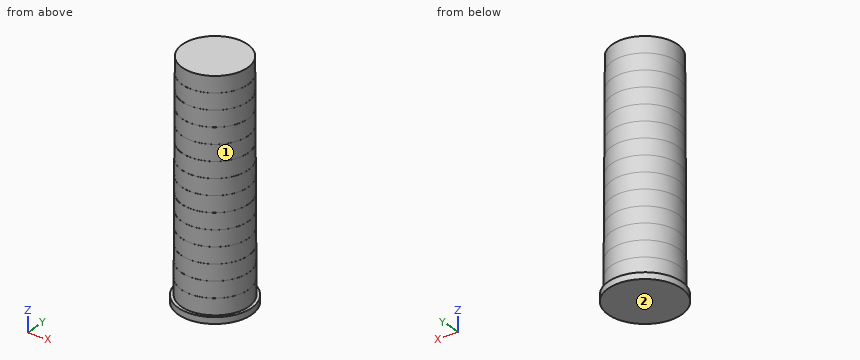
from build123d import *

# Parameters (mm, degrees)
F0_R      = 21.1
F1_DEPTH  = 10
F2_R      = 21.05
F3_DEPTH  = 10
F4_R      = 21
F5_DEPTH  = 10
F6_R      = 20.95
F7_DEPTH  = 10
F8_R      = 23
F8_R_2    = 21.1
F9_DEPTH  = 4
F10_R     = 20.9
F11_DEPTH = 10
F12_R     = 20.85
F13_DEPTH = 10
F14_R     = 20.8
F15_DEPTH = 10
F16_R     = 20.75
F17_DEPTH = 10
F18_R     = 20.7
F19_DEPTH = 10
F20_R     = 20.65
F21_DEPTH = 10
F22_R     = 20.6
F23_DEPTH = 10
F24_R     = 20.55
F25_DEPTH = 10
F26_R     = 20.5
F27_DEPTH = 10
F28_R     = 20.45
F29_DEPTH = 10


with BuildPart() as f1:
    # F0 (on Top) → F1 (new body)
    with BuildSketch(Plane.XY):
        Circle(F0_R)
    extrude(amount=F1_DEPTH)

    # F2 (on face) → F3 (join)
    with BuildSketch(Plane.XY.offset(10)):
        Circle(F2_R)
    extrude(amount=F3_DEPTH)

    # F4 (on face) → F5 (join)
    with BuildSketch(Plane.XY.offset(20)):
        Circle(F4_R)
    extrude(amount=F5_DEPTH)

    # F6 (on face) → F7 (join)
    with BuildSketch(Plane.XY.offset(30)):
        Circle(F6_R)
    extrude(amount=F7_DEPTH)

    # F8 (on face) → F9 (join)
    with BuildSketch(Plane(origin=(0, 0, 0), x_dir=(1, 0, 0), z_dir=(0, 0, -1))):
        Circle(F8_R)
        Circle(F8_R_2, mode=Mode.SUBTRACT)
        Circle(F8_R_2)
    extrude(amount=F9_DEPTH)

    # F10 (on face) → F11 (join)
    with BuildSketch(Plane.XY.offset(40)):
        Circle(F10_R)
    extrude(amount=F11_DEPTH)

    # F12 (on face) → F13 (join)
    with BuildSketch(Plane.XY.offset(50)):
        Circle(F12_R)
    extrude(amount=F13_DEPTH)

    # F14 (on face) → F15 (join)
    with BuildSketch(Plane.XY.offset(60)):
        Circle(F14_R)
    extrude(amount=F15_DEPTH)

    # F16 (on face) → F17 (join)
    with BuildSketch(Plane.XY.offset(70)):
        Circle(F16_R)
    extrude(amount=F17_DEPTH)

    # F18 (on face) → F19 (join)
    with BuildSketch(Plane.XY.offset(80)):
        Circle(F18_R)
    extrude(amount=F19_DEPTH)

    # F20 (on face) → F21 (join)
    with BuildSketch(Plane.XY.offset(90)):
        Circle(F20_R)
    extrude(amount=F21_DEPTH)

    # F22 (on face) → F23 (join)
    with BuildSketch(Plane.XY.offset(100)):
        Circle(F22_R)
    extrude(amount=F23_DEPTH)

    # F24 (on face) → F25 (join)
    with BuildSketch(Plane.XY.offset(110)):
        Circle(F24_R)
    extrude(amount=F25_DEPTH)

    # F26 (on face) → F27 (join)
    with BuildSketch(Plane.XY.offset(120)):
        Circle(F26_R)
    extrude(amount=F27_DEPTH)

    # F28 (on face) → F29 (join)
    with BuildSketch(Plane.XY.offset(130)):
        Circle(F28_R)
    extrude(amount=F29_DEPTH)


solid = f1.part
CAD build for the part. Positions are in the model's coordinates, mm. Face numbers are marked on the shaded views. A direction names the side the tool comes from. Round coordinates to 2 decimals unless told otherwise and drop trailing zeros. Write each loop counter-clockwise with the first axis right and the second up, starting at its lowest first coordinate (ties: lowest second). Pieces come first, ordered by that corner, then holes.
(1) 3-axis set-ups, long thin cutter, end or side, ignore diameter. For the marked faces 1 and 2: which of +Z, -Z, +X, -X, +Y, -Y reach the whole face in a straight line?
(2) Drop flat-ended pins along their axis: P1, Ø3, axis at x = -17.5, z = 77.5, coming from the +Y side; P2, Ø8, axis at y = -1, z = 87, coming from the -X side; P3, Ø8, axis at y = 2.5, z = 58, coming from the +X side. Give the stop position or say it passes through.
(3) Slice it at A-A, the plane z = 93.5. Write the cut outline in (x, y), and give its area (3 significant figures).
(4) Probe line 1 along Y through (x, z) = (-2, 15.5); line 2 along X through (y, z) = (-2.5, 84.5). List the from-to ranges inside material, lowest first.
From the geometry:
1. face 1: +Z
1. face 2: -Z, +X, -X, +Y, -Y
2. P1: stops at y = 13.21
2. P2: stops at x = -20.7
2. P3: stops at x = 20.85
3. outline: circle Ø41.3 at (0, 0)
3. area: 1,340 mm2
4. line 1: y = -20.95 to 20.95
4. line 2: x = -20.55 to 20.55
